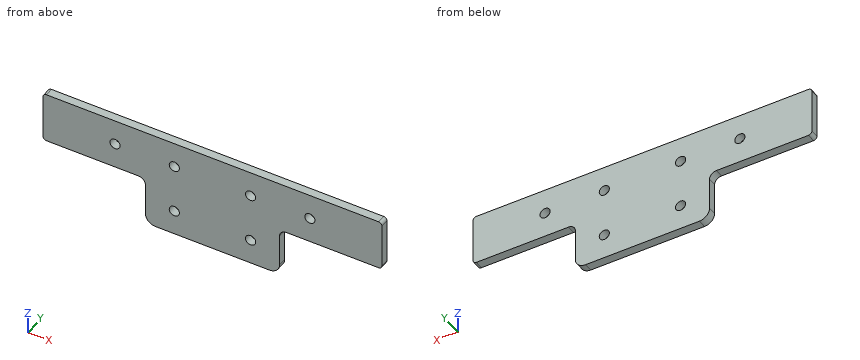
from build123d import *

# Parameters (mm, degrees)
SKETCH1_W           = 127
SKETCH1_H           = 19.05
BOSS_EXTRUDE1_DEPTH = 3.175
SKETCH3_W           = 50.292
SKETCH3_H           = 18.288
BOSS_EXTRUDE2_DEPTH = 3.175
SKETCH2_R           = 1.905
CUT_EXTRUDE1_DEPTH  = 4.175
FILLET1_R           = 1.27
FILLET2_R           = 2.54
FILLET3_R           = 3.81


with BuildPart() as part:
    # Sketch1 → Boss-Extrude1 (new body)
    with BuildSketch(Plane(origin=(0, 0, 0), x_dir=(1, 0, 0), z_dir=(0, 1, 0))):
        Rectangle(SKETCH1_W, SKETCH1_H)
    extrude(amount=BOSS_EXTRUDE1_DEPTH)

    # Sketch3 → Boss-Extrude2 (add, through all)
    with BuildSketch(Plane(origin=(0, 3.175, 0), x_dir=(1, 0, 0), z_dir=(0, 1, 0))):
        with Locations((0, 18.669)):
            Rectangle(SKETCH3_W, SKETCH3_H)
    extrude(amount=-BOSS_EXTRUDE2_DEPTH)

    # Sketch2 → Cut-Extrude1 (cut, through all)
    with BuildSketch(Plane(origin=(0, 3.175, 0), x_dir=(1, 0, 0), z_dir=(0, 1, 0))):
        with Locations((-36.5125, 0)):
            Circle(SKETCH2_R)
        with Locations((36.5125, 0)):
            Circle(SKETCH2_R)
        with Locations((-14.2875, 0)):
            Circle(SKETCH2_R)
        with Locations((14.2875, 0)):
            Circle(SKETCH2_R)
        with Locations((-14.2875, 18.415)):
            Circle(SKETCH2_R)
        with Locations((14.2875, 18.415)):
            Circle(SKETCH2_R)
    extrude(amount=-CUT_EXTRUDE1_DEPTH, mode=Mode.SUBTRACT)

    # Fillet1
    fillet1_edges = [part.edges().sort_by_distance(p)[0] for p in [
        (63.5, 1.5875, 9.525),
        (-63.5, 1.5875, 9.525),
        (-63.5, 1.5875, -9.525),
        (63.5, 1.5875, -9.525),
    ]]
    fillet(fillet1_edges, radius=FILLET1_R)

    # Fillet2
    fillet2_edges = [part.edges().sort_by_distance(p)[0] for p in [
        (-25.146, 1.5875, -9.525),
        (25.146, 1.5875, -9.525),
    ]]
    fillet(fillet2_edges, radius=FILLET2_R)

    # Fillet3
    fillet3_edges = [part.edges().sort_by_distance(p)[0] for p in [
        (-25.146, 1.5875, -27.813),
        (25.146, 1.5875, -27.813),
    ]]
    fillet(fillet3_edges, radius=FILLET3_R)


solid = part.part
The model under review builds one solid part; all positions refer to its coordinate system, in mm. Coordinates: 2 decimals unless noted, no trailing zeros. Write each loop counter-clockwise with the first axis right and the second up, starting at its lowest first coordinate (ties: lowest second). Pieces come first, ordered by that corner, then holes. Notation, with made-up numbers: (48, -23) - (89, -23) arc R20 ccw to (89, -7) - close; hole circle Ø9 at (66, 22). An arc over 180 degrees is marked (long way). Answer as a JSON object with one key per item and string values. Group by question number.
1. To check wall thickness, follow probe 1 along X at (y, z) = (2.35, 0); probe 2 along Z at (x, y) = (15.5, 2.25) (3 decimals); probe 3 along X at (y, z) = (0.2, -17.5). State the ranges of each line that lie inside material, in increasing order.
2. Clearance check with flat-ended pins moving along their axes: pin 1 Ø1.6 at (y, z) = (1.5, -15) entering from +X; pin 2 Ø1.5 at (x, y) = (30.5, 2) entering from -Z (3 decimals); pin 3 Ø6 at (x, z) = (36.51, 0) entering from -Y; pin 4 Ø1 at (y, z) = (1, -20) entering from -X. State where each tip first meets the part, or that it passes through.
3. Add section A-A (z = 0). Give the boundary of the cut face in (x, y) (1 decimal), plus the area to 3 significant figures.
4. Add section B-B (y = 2.3). Give the boundary of the cut face in (x, z) (1 decimal), plus the area to 3 significant figures.
Findings:
{
 "1": {"probe 1": "-63.5 to -38.42, -34.61 to -16.19, -12.38 to 12.38, 16.19 to 34.61, 38.42 to 63.5", "probe 2": "-27.813 to -19.884, -16.946 to -1.469, 1.469 to 9.525", "probe 3": "-25.15 to -15.96, -12.62 to 12.62, 15.96 to 25.15"},
 "2": {"pin 1": "x = 25.15", "pin 2": "z = -9.525", "pin 3": "y = 0", "pin 4": "x = -25.15"},
 "3": {"outline": "(-63.5, 0) - (-38.4, 0) - (-38.4, 3.2) - (-63.5, 3.2) - close; (-34.6, 0) - (-16.2, 0) - (-16.2, 3.2) - (-34.6, 3.2) - close; (-12.4, 0) - (12.4, 0) - (12.4, 3.2) - (-12.4, 3.2) - close; (16.2, 0) - (34.6, 0) - (34.6, 3.2) - (16.2, 3.2) - close; (38.4, 0) - (63.5, 0) - (63.5, 3.2) - (38.4, 3.2) - close", "area": "355 mm²"},
 "4": {"outline": "(-63.5, -8.3) arc R1.3 ccw to (-62.2, -9.5) - (-27.7, -9.5) arc R2.5 cw to (-25.1, -12.1) - (-25.1, -24) arc R3.8 ccw to (-21.3, -27.8) - (21.3, -27.8) arc R3.8 ccw to (25.1, -24) - (25.1, -12.1) arc R2.5 cw to (27.7, -9.5) - (62.2, -9.5) arc R1.3 ccw to (63.5, -8.3) - (63.5, 8.3) arc R1.3 ccw to (62.2, 9.5) - (-62.2, 9.5) arc R1.3 ccw to (-63.5, 8.3) - close; hole circle Ø3.8 at (-36.5, 0); hole circle Ø3.8 at (-14.3, -18.4); hole circle Ø3.8 at (-14.3, 0); hole circle Ø3.8 at (14.3, -18.4); hole circle Ø3.8 at (14.3, 0); hole circle Ø3.8 at (36.5, 0)", "area": "3,270 mm²"}
}
